Autodesk Inventor part; units mm, degrees
ref_plane "YZ Plane" through (0, 0, 0) normal (1, 0, 0) x (0, 1, 0)
ref_plane "XZ Plane" through (0, 0, 0) normal (0, 1, 0) x (-1, 0, 0)
ref_plane "XY Plane" through (0, 0, 0) normal (0, 0, 1) x (1, 0, 0)
sketch "Sketch1" plane through (0, 0, 0) normal (0, 0, 1) x (1, 0, 0)
  point P0 (0, 0)
sketch "Sketch2" plane through (0, 0, 0) normal (0, 0, 1) x (1, 0, 0)
  line L0 (0, 0) -> (170, 0)
  line L1 (170, 0) -> (170, 10)
  line L2 (170, 10) -> (0, 10)
  line L3 (0, 10) -> (0, 0)
  circle A0 centre (165, 5) radius 2.5
  circle A1 centre (45, 5) radius 2.5
  line L4 (45, 2.5) -> (165, 2.5)
  line L5 (165, 2.5) -> (165, 7.5)
  line L6 (165, 7.5) -> (45, 7.5)
  line L7 (45, 7.5) -> (45, 2.5)
  point P0 (45, 7.5)
  point P1 (165, 2.5)
  dimension "d4" = 5
  dimension "d5" = 5
  dimension "d0" = 170
  dimension "d1" = 10
  dimension "d2" = 5
  dimension "d3" = 5
  dimension "d6" = 120
  dimension "d7" = 5
  dimension "d8" = 2.5
  dimension "d9" = 2.5
extrude "Extrusion1" add sketch "Sketch2" along normal blind 50
sketch "Sketch3" plane through (0, 10, 0) normal (0, 1, 0) x (1, 0, 0)
  line L0 (170, 0) -> (170, -50)
  line L1 (170, -45) -> (-20, -45)
  line L2 (-20, -45) -> (-20, -5)
  line L3 (-20, -5) -> (170, -5)
  line L4 (170, -5) -> (170, -45)
  line L5 (170, -50) -> (0, -50)
  line L6 (170, 0) -> (0, 0)
  dimension "d12" = 190
  dimension "d13" = 5
  dimension "d14" = 5
extrude "Extrusion2" cut sketch "Sketch3" against normal blind 10
sketch "Sketch4" plane through (0, 0, 0) normal (0, 0, -1) x (-1, 0, 0)
  circle A0 centre (-20, 5) radius 2.5
  line L0 (0, 10) -> (0, 0)
  line L1 (0, 0) -> (-170, 0)
  dimension "d17" = 20
  dimension "d18" = 5
  dimension "d19" = 5
extrude "Extrusion3" add sketch "Sketch4" along normal blind 1 and the other way blind 50
properties part number "Base"
CAD build for the part. Positions are in the model's coordinates, mm. A direction names the side the tool comes from. Coordinates: 2 decimals unless noted, no trailing zeros. Order: outer loops, then holes, each group sorted by start corner. A loop starts at its lowest first (then second) coordinate and runs counter-clockwise, first axis right, second up. Notation, with made-up numbers: M 56.25,13.5 L 103.25,13.5 A14 ccw 103.25,36.5 Z; hole C -22,50 d1. An arc over 180 degrees is marked long. Answer as CSV lines item,"result".
1) Cut at B-B (x = 26). List the corners of the cut face in (y, z).
Verdict:
outline,"M 0,0 L 10,0 L 10,5 L 0,5 Z; M 0,45 L 10,45 L 10,50 L 0,50 Z"
2) Cut at A-A (y = 5). List the corners of the cut face in (x, z), then the cut area to 3 significant figures.
Verdict:
outline,"M 0,0 L 17.5,0 L 17.5,-1 L 22.5,-1 L 22.5,0 L 42.5,0 L 42.5,5 L 22.5,5 L 22.5,45 L 42.5,45 L 42.5,50 L 0,50 L 0,45 L 17.5,45 L 17.5,5 L 0,5 Z; M 167.5,0 L 170,0 L 170,5 L 167.5,5 Z; M 167.5,45 L 170,45 L 170,50 L 167.5,50 Z"
area,"655 mm2"
3) 3-axis set-ups, long thin cutter, end or side, ignore diameter. For faces 1 (the cylindrical face through (22.5, 5.1, 24.7)), 2 (the cylindrical face through (22.5, 4.9, -0.5)), 3 (the cylindrical face through (42.5, 4.9, 2.5)): which of +Z, -Z, +X, -X, +Y, -Y reach the whole face in a straight line?
Verdict:
face 1,"none"
face 2,"-Z"
face 3,"+Z, -Z"
4) Flat gauge pins, fed straight in: P1, Ø5.5, axis at x = 119, z = 46.5, coming from the -Y side; P2, Ø3, axis at x = 105.5, y = 3.5, coming from the -Z side; P3, Ø5, axis at y = 2, z = 19.5, coming from the +X side; P4, Ø1, axis at x = 57, y = 5.5, coming from the -Z side. Where does each tip first touch, or does it go through?
Verdict:
P1,"y = 0"
P2,"z = 0"
P3,"x = 22.45"
P4,"through"
5) Cut at D-D (z = 11). List the corners of the cut face in (x, y), then the cut area to 3 significant figures.
Verdict:
outline,"C 20,5 d5"
area,"19.6 mm2"
6) Cut at C-C (x = 70.5). List the corners of the cut face in (y, z), then the cut area to 3 significant figures.
Verdict:
outline,"M 0,0 L 2.5,0 L 2.5,5 L 0,5 Z; M 0,45 L 2.5,45 L 2.5,50 L 0,50 Z; M 7.5,0 L 10,0 L 10,5 L 7.5,5 Z; M 7.5,45 L 10,45 L 10,50 L 7.5,50 Z"
area,"50.0 mm2"
7) Mould opens along X. For faces 4 (the flat face through (65, 8, 50)), 5 (the flat face through (170, 5, 47)), 6 (the flat face through (106, 7.5, 2)) say: released by +X, released by -X, zero draft, split by the parting line, or undercut.
Verdict:
face 4,"zero draft"
face 5,"released by +X"
face 6,"undercut"
8) Drill centre lines: L1, parallel to Z at x = 10, y = 3.75; L2, parallel to Y at x = 48.5, z = 47; L3, parallel to X at y = 4.75, z = 28.5. Where is each one in solid material? Low to high. Write a range as from..to.
Verdict:
L1,"0..5, 45..50"
L2,"0..2.5, 7.5..10"
L3,"17.51..22.49"
